```python
from build123d import *

# Parameters (mm, degrees)
SKETCH1_R           = 57.5
BOSS_EXTRUDE1_DEPTH = 4.5
SKETCH2_W           = 140
SKETCH2_H           = 70
BOSS_EXTRUDE2_DEPTH = 4.5
BOSS_EXTRUDE3_DEPTH = 4.5
SKETCH4_R           = 43
CUT_EXTRUDE1_DEPTH  = 5.5
SKETCH7_R           = 3.25
CUT_EXTRUDE8_DEPTH  = 5.5
LPATTERN1_COUNT     = 3
LPATTERN1_PITCH     = 20
CUT_EXTRUDE5_START  = -1
SKETCH5_R           = 2.25
CUT_EXTRUDE5_DEPTH  = 6.5
CIRPATTERN1_COUNT   = 12
SKETCH12_R          = 3.5
CUT_EXTRUDE17_DEPTH = 5.5
CIRPATTERN2_COUNT   = 4
SKETCH13_R          = 3.25
CUT_EXTRUDE18_DEPTH = 10
LPATTERN2_COUNT     = 3
LPATTERN2_PITCH     = 20


with BuildPart() as part:
    # Sketch1 → Boss-Extrude1 (new body)
    with BuildSketch(Plane(origin=(0, 0, 0), x_dir=(1, 0, 0), z_dir=(0, 1, 0))):
        Circle(SKETCH1_R)
    extrude(amount=BOSS_EXTRUDE1_DEPTH)

    # Sketch2 → Boss-Extrude2 (add)
    with BuildSketch(Plane(origin=(0, 0, 0), x_dir=(1, 0, 0), z_dir=(0, 1, 0))):
        with Locations((63.125798099, 0)):
            Rectangle(SKETCH2_W, SKETCH2_H)
    extrude(amount=BOSS_EXTRUDE2_DEPTH)

    # Sketch3 → Boss-Extrude3 (add)
    with BuildSketch(Plane(origin=(0, 0, 0), x_dir=(1, 0, 0), z_dir=(0, 1, 0))):
        Polygon((89.373258538, 35), (13.76852627, 55.827212758), (13.76852627, 13.558751548), align=None)
    extrude(amount=BOSS_EXTRUDE3_DEPTH)

    # Sketch4 → Cut-Extrude1 (cut, through all)
    with BuildSketch(Plane(origin=(0, 4.5, 0), x_dir=(1, 0, 0), z_dir=(0, 1, 0))):
        Circle(SKETCH4_R)
    extrude(amount=-CUT_EXTRUDE1_DEPTH, mode=Mode.SUBTRACT)

    # Sketch7 → Cut-Extrude8 (cut, through all)
    with BuildSketch(Plane(origin=(0, 4.5, 0), x_dir=(1, 0, 0), z_dir=(0, 1, 0))):
        with Locations((123.125798099, 15)):
            Circle(SKETCH7_R)
        with Locations((123.125798099, -15)):
            Circle(SKETCH7_R)
    cut_extrude8 = extrude(amount=-CUT_EXTRUDE8_DEPTH, mode=Mode.SUBTRACT)

    # LPattern1: Cut-Extrude8 ×3
    with Locations(*[(-i * LPATTERN1_PITCH, 0, 0) for i in range(1, LPATTERN1_COUNT)]):
        add(cut_extrude8, mode=Mode.SUBTRACT)

    # Sketch5 → Cut-Extrude5 (cut)
    with BuildSketch(Plane(origin=(0, 0, 0), x_dir=(1, 0, 0), z_dir=(0, 1, 0)).offset(CUT_EXTRUDE5_START)):
        with Locations((-51, 0)):
            Circle(SKETCH5_R)
    cut_extrude5 = extrude(amount=CUT_EXTRUDE5_DEPTH, mode=Mode.SUBTRACT)

    # CirPattern1: Cut-Extrude5 ×12 about axis
    cirpattern1_axis = Axis((0, 0, 0), (0, 1, 0))
    for i in range(1, CIRPATTERN1_COUNT):
        add(cut_extrude5.rotate(cirpattern1_axis, i * 360 / CIRPATTERN1_COUNT), mode=Mode.SUBTRACT)

    # Sketch12 → Cut-Extrude17 (cut, through all)
    with BuildSketch(Plane(origin=(0, 4.5, 0), x_dir=(1, 0, 0), z_dir=(0, 1, 0))):
        with Locations((-49.262217141, 13.1997713)):
            Circle(SKETCH12_R)
    cut_extrude17 = extrude(amount=-CUT_EXTRUDE17_DEPTH, mode=Mode.SUBTRACT)

    # CirPattern2: Cut-Extrude17 ×4 about axis
    cirpattern2_axis = Axis((0, 0, 0), (0, 1, 0))
    for i in range(1, CIRPATTERN2_COUNT):
        add(cut_extrude17.rotate(cirpattern2_axis, i * 360 / CIRPATTERN2_COUNT), mode=Mode.SUBTRACT)

    # Sketch13 → Cut-Extrude18 (cut)
    with BuildSketch(Plane(origin=(0, 4.5, 0), x_dir=(1, 0, 0), z_dir=(0, 1, 0))):
        with Locations((123.125798099, 0)):
            Circle(SKETCH13_R)
    cut_extrude18 = extrude(amount=-CUT_EXTRUDE18_DEPTH, mode=Mode.SUBTRACT)

    # LPattern2: Cut-Extrude18 ×3
    with Locations(*[(-i * LPATTERN2_PITCH, 0, 0) for i in range(1, LPATTERN2_COUNT)]):
        add(cut_extrude18, mode=Mode.SUBTRACT)


solid = part.part
```
Build history of the part. All positions in model axes, mm. A direction names the side the tool comes from. Coordinates: 2 decimals unless noted, no trailing zeros. Write each loop counter-clockwise with the first axis right and the second up, starting at its lowest first coordinate (ties: lowest second). Pieces come first, ordered by that corner, then holes.
1. Drill centre lines: probe 1 along Z at (x, y) = (27.5, 2.8); probe 2 along X at (y, z) = (3.4, -15); probe 3 along X at (y, z) = (1.7, 15). Where is each one in solid material? Low to high.
Answer block:
probe 1: z = -52.04 to -45.2, -43.14 to -33.06, 33.06 to 43.14, 45.2 to 50.5
probe 2: x = -55.51 to -52.26, -46.26 to -40.3, 40.3 to 79.88, 86.38 to 99.88, 106.38 to 119.88, 126.38 to 133.13
probe 3: x = -55.51 to -40.3, 40.3 to 46.26, 52.26 to 79.88, 86.38 to 99.88, 106.38 to 119.88, 126.38 to 133.13
2. 3-axis set-ups, long thin cutter, end or side, ignore diameter. For faces 4 (the flat face through (111, 2, -35)), 5 (the cylindrical face through (23.842, 2.218, -45.688)): which of +Z, -Z, +X, -X, +Y, -Y reach the whole face in a straight line?
Answer block:
face 4: -Z, +X, +Y, -Y
face 5: +Y, -Y
3. Band-saw the part on C-C, the plane z = 31.5. Give the cut face in (x, y).
Answer block:
outline: (-48.1, 0) - (-29.27, 0) - (-29.27, 4.5) - (-48.1, 4.5) - close; (29.27, 0) - (133.13, 0) - (133.13, 4.5) - (29.27, 4.5) - close
4. Drop a flat-ended pin along its axis: pin 1 (2 mm diameter, centred on x = 98, y = 2, fed in from +Z). Give the stop position or say it passes through.
Answer block:
pin 1: stops at z = 35
5. Band-saw the part on D-D, the plane x = 78. Give the cut face in (y, z).
Answer block:
outline: (0, -38.13) - (4.5, -38.13) - (4.5, 35) - (0, 35) - close
6. Band-saw the part on B-B, the plane y = 2.6. Give the number of separate pieces and of enclosed holes in the cut face, and give its area (3 significant figures).
Answer block:
separate pieces: 1
enclosed holes: 26
area: 9,870 mm2
7. Band-saw the part on A-A, the plane x = 40. Give the cut face in (y, z), and give its area (3 significant figures).
Answer block:
outline: (0, -48.6) - (4.5, -48.6) - (4.5, -15.78) - (0, -15.78) - close; (0, 15.78) - (4.5, 15.78) - (4.5, 41.31) - (0, 41.31) - close
area: 263 mm2
8. Pull direction X, two halves, no side cores. Call faces 1 (the flat face through (89, 2, 35)), 2 (the cylindrical face through (46.4, 2.22, 25.21)), 3 (the flat face through (53.58, 2.22, -44.86)): released by +X, released by -X, zero draft, split by the parting line, or undercut.
Answer block:
face 1: zero draft
face 2: undercut
face 3: released by +X
